Autodesk Inventor part; units mm, degrees
ref_plane "YZ Plane" through (0, 0, 0) normal (1, 0, 0) x (0, 1, 0)
ref_plane "XZ Plane" through (0, 0, 0) normal (0, 1, 0) x (-1, 0, 0)
ref_plane "XY Plane" through (0, 0, 0) normal (0, 0, 1) x (1, 0, 0)
sketch "スケッチ1" plane through (0, 0, 0) normal (0, 1, 0) x (-1, 0, 0)
  line L0 (-15, -15) -> (15, -15)
  line L1 (15, -15) -> (15, 15)
  line L2 (15, 15) -> (-15, 15)
  line L3 (-15, 15) -> (-15, -15)
  line L4 (-15, -15) -> (15, 15) construction
  line L5 (15, -15) -> (-15, 15) construction
  circle A0 centre (0, 0) radius 4
  dimension "d0" = 30
  dimension "d1" = 30
  dimension "d2" = 8
extrude "押し出し1" add sketch "スケッチ1" along normal blind 0.8
sketch "スケッチ2" plane through (0, 0.8, 0) normal (0, 1, 0) x (1, 0, 0)
  circle A0 centre (-12.5, -12.5) radius 1.6
  line L0 (0, -18.82) -> (0, 21.247)
  line L1 (-16.0432, 0) -> (16.9483, 0)
  circle A1 centre (-12.5, 12.5) radius 1.6
  circle A2 centre (12.5, -12.5) radius 1.6
  circle A3 centre (12.5, 12.5) radius 1.6
  line L2 (-15, 15) -> (-15, -15)
  line L3 (-15, -15) -> (15, -15)
  point P0 (0, 0)
  dimension "d5" = 3.2
  dimension "d10" = 25
  dimension "d13" = 25
  dimension "d18" = 2.5
  dimension "d19" = 2.5
extrude "押し出し2" cut sketch "スケッチ2" against normal through all contours A0 | A1 | A2 | A3
properties part number "Base"
Can you work these out from the model? Positions are in its coordinate system, mm. Coordinates: 2 decimals unless noted, no trailing zeros. Order: outer loops, then holes, each group sorted by start corner. A loop starts at its lowest first (then second) coordinate and runs counter-clockwise, first axis right, second up. Notation, with made-up numbers: M 47,37.5 L 97,37.5 A11 ccw 97,48.5 Z; hole C 25,41.25 d7. An arc over 180 degrees is marked long. Answer as CSV lines item,"result".
(1) Suppose I cut it at C-C on x = 12.5. Please give me the cut outline in (y, z), plus the area to 3 significant figures.
Geometry check:
outline,"M 0,-15 L 0.8,-15 L 0.8,-14.1 L 0,-14.1 Z; M 0,-10.9 L 0.8,-10.9 L 0.8,10.9 L 0,10.9 Z; M 0,14.1 L 0.8,14.1 L 0.8,15 L 0,15 Z"
area,"18.9 mm^2"
(2) Please list where these lines run through material, in increasing order: L1, parallel to X at y = 0.6, z = 12.5; L2, parallel to Z at x = 12, y = 0.55.
Geometry check:
L1,"-15 to -14.1, -10.9 to 10.9, 14.1 to 15"
L2,"-15 to -14.02, -10.98 to 10.98, 14.02 to 15"
(3) If we mould it in two halves opening along Y, with no side actions, what happens to faces 1 (the cylindrical face through (10.9, 0.41, -12.57)), 2 (the flat face through (4, 0, 4)), 3 (the flat face through (4, 0.8, 4))? For each: released by +Y, released by -Y, zero draft, split by the parting line, or undercut.
Geometry check:
face 1,"zero draft"
face 2,"released by -Y"
face 3,"released by +Y"
(4) Suppose I cut it at B-B on y = 0.6. Please give me the cut outline in (x, z), plus the area to 3 significant figures.
Geometry check:
outline,"M -15,-15 L 15,-15 L 15,15 L -15,15 Z; hole C -12.5,-12.5 d3.2; hole C -12.5,12.5 d3.2; hole C 0,0 d8; hole C 12.5,-12.5 d3.2; hole C 12.5,12.5 d3.2"
area,"818 mm^2"
(5) I'm going to push a flat-ended pin straight in: pin 1 (7 mm diameter, centred on x = 0, z = 0, fed in from +Y). Where does the tip first touch, or does it pass through?
Geometry check:
pin 1,"through"
(6) Suppose I cut it at A-A on x = 0. Please give me the cut outline in (y, z), plus the area to 3 significant figures.
Geometry check:
outline,"M 0,-15 L 0.8,-15 L 0.8,-4 L 0,-4 Z; M 0,4 L 0.8,4 L 0.8,15 L 0,15 Z"
area,"17.6 mm^2"
(7) Suppose I cut it at D-D on z = 2.5. Please give me the cut outline in (x, y).
Geometry check:
outline,"M -15,0 L -3.12,0 L -3.12,0.8 L -15,0.8 Z; M 3.12,0 L 15,0 L 15,0.8 L 3.12,0.8 Z"
